Work out the finished part from the listing and answer in its coordinate system (mm). Face numbers are marked on the shaded views. Round coordinates to 2 decimals unless told otherwise and drop trailing zeros. Write each loop counter-clockwise with the first axis right and the second up, starting at its lowest first coordinate (ties: lowest second). Pieces come first, ordered by that corner, then holes.
1. Straight lines are drawn through the part: probe 1 along Y at (x, z) = (136.5, 6.25); probe 2 along X at (y, z) = (21.5, 7.5); probe 3 along Y at (x, z) = (26.5, 6.75). For each, find the intervals that lie inside material, in ascending order.
2. Find section C-C (y = -53.5). Write down the section's boundary in (x, z), and give its area (3 significant figures).
3. A flat-ended cylindrical pin translates along its axis: pin 1 Ø1.5 at (x, y) = (-152.5, 35) entering from +Z. Find the tip coordinate at first contact, or state that the pin passes through.
4. Find section D-D (x = 143.5). Write down the section's boundary in (y, z), and give its area (3 significant figures).
5. Find section B-B (z = 7). Write down the section's boundary in (x, y).
6. Find section A-A (x = -108). Write down the section's boundary in (y, z), and give its area (3 significant figures).
7. Determine the mould class of the marked faces 1 and 2 for opening direction Y: pulls with the +Y half, pulls with the -Y half, needs draft (parallel to the pull), parting line crosses it, or undercut.
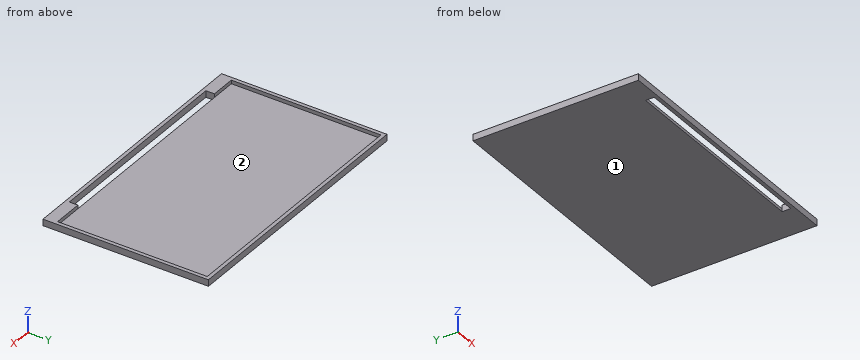
Autodesk Fusion 360 part; units mm, degrees
sketch "Szkic1" plane through (0, 0, 0) normal (0, 0, 1) x (1, 0, 0)
  line L0 (-190.7916, 55) -> (169.2084, 55)
  line L1 (169.2084, 55) -> (169.2084, -153)
  line L2 (169.2084, -153) -> (-190.7916, -153)
  line L3 (-190.7916, -153) -> (-190.7916, 55)
  line L4 (-186.2916, 51.8) -> (159.7084, 51.8)
  line L5 (159.7084, 51.8) -> (159.7084, -145.2)
  line L6 (159.7084, -145.2) -> (-186.2916, -145.2)
  line L7 (-186.2916, -145.2) -> (-186.2916, 51.8)
  line L8 (-155.7916, -153) -> (127.2084, -153)
  line L9 (127.2084, -153) -> (127.2084, -164.9)
  line L10 (127.2084, -164.9) -> (-155.7916, -164.9)
  line L11 (-155.7916, -164.9) -> (-155.7916, -153)
  line L12 (-195.7916, 60) -> (174.2084, 60)
  line L13 (174.2084, 60) -> (174.2084, -169.9)
  line L14 (174.2084, -169.9) -> (-195.7916, -169.9)
  line L15 (-195.7916, -169.9) -> (-195.7916, 60)
  dimension "d1" = 360
  dimension "d2" = 208
  dimension "d3" = 346
  dimension "d4" = 197
  dimension "d5" = 9.5
  dimension "d6" = 7.8
  dimension "d7" = 11.9
  dimension "d8" = 35
  dimension "d9" = 283
  dimension "d10" = 370
  dimension "d11" = 5
  dimension "d12" = 5
  dimension "d13" = 5
extrude "Wyciągnięcie proste1" add sketch "Szkic1" along normal blind 5 contours L12 L13 L14 L15
extrude "Wyciągnięcie proste2" add 1 faces at (156.8751, -162.6, 5) along direction (0, 0, 1) blind 4
extrude "Wyciągnięcie proste3" add sketch "Szkic1" along normal blind 4 contours L0 L1 L2 L3 L8 | L4 L5 L6 L7
Worked answers:
1. probe 1: y = -169.9 to -153, 55 to 60
1. probe 2: x = -195.79 to -190.79, 169.21 to 174.21
1. probe 3: y = -169.9 to -164.9, 55 to 60
2. outline: (-195.79, 0) - (174.21, 0) - (174.21, 9) - (169.21, 9) - (169.21, 4) - (-190.79, 4) - (-190.79, 9) - (-195.79, 9) - close
2. area: 1,530 mm2
3. pin 1: stops at z = 4
4. outline: (-169.9, 0) - (60, 0) - (60, 9) - (55, 9) - (55, 4) - (-153, 4) - (-153, 9) - (-169.9, 9) - close
4. area: 1,030 mm2
5. outline: (-195.79, -169.9) - (174.21, -169.9) - (174.21, 60) - (-195.79, 60) - close; hole (-190.79, -153) - (-155.79, -153) - (-155.79, -164.9) - (127.21, -164.9) - (127.21, -153) - (169.21, -153) - (169.21, 55) - (-190.79, 55) - close
6. outline: (-169.9, 0) - (-164.9, 0) - (-164.9, 9) - (-169.9, 9) - close; (-153, 0) - (60, 0) - (60, 9) - (55, 9) - (55, 4) - (-153, 4) - close
6. area: 922 mm2
7. face 1: needs draft
7. face 2: undercut
